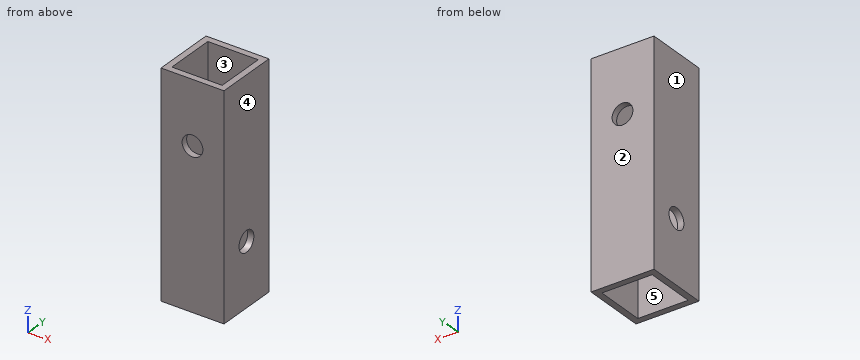
Autodesk Inventor part; units mm, degrees
ref_plane "YZ Plane" through (0, 0, 0) normal (1, 0, 0) x (0, 1, 0)
ref_plane "XZ Plane" through (0, 0, 0) normal (0, 1, 0) x (-1, 0, 0)
ref_plane "XY Plane" through (0, 0, 0) normal (0, 0, 1) x (1, 0, 0)
sketch "スケッチ1" plane through (0, 0, 0) normal (0, 0, 1) x (1, 0, 0)
  line L0 (5, -5) -> (-5, -5)
  line L1 (-5, -5) -> (-5, 5)
  line L2 (-5, 5) -> (5, 5)
  line L3 (5, 5) -> (5, -5)
  line L4 (5, -5) -> (-5, 5) construction
  line L5 (-5, -5) -> (5, 5) construction
  line L6 (4, 4) -> (-4, 4)
  line L7 (-4, 4) -> (-4, -4)
  line L8 (-4, -4) -> (4, -4)
  line L9 (4, -4) -> (4, 4)
  point P0 (0, 0)
  dimension "d0" = 10
  dimension "d1" = 10
  dimension "d2" = 1
extrude "押し出し1" add sketch "スケッチ1" along normal blind 35
sketch "スケッチ2" plane through (5, -5, 0) normal (1, 0, 0) x (0, 0, -1)
  line L0 (-35, 9) -> (-35, 1)
  line L1 (-35, 5) -> (0, 5)
  line L2 (0, 9) -> (0, 1)
  point P0 (-10, 5)
  dimension "d5" = 10
hole "穴1" at (5, 0, 10) direction (-1, 0, 0) diameter 3.3 end through all
sketch "スケッチ3" plane through (-5, 5, 0) normal (0, 1, 0) x (1, 0, 0)
  line L0 (5, 0) -> (5, -35)
  line L1 (0, -35) -> (10, -35)
  line L2 (10, 0) -> (0, 0)
  point P0 (5, -25)
  dimension "d13" = 25
hole "穴2" at (0, 5, 25) direction (0, -1, 0) diameter 3.3 end through all
properties part number "small_kaku_1010_santen_1020"
For this review, take the finished solid that the model builds, in its own axes (mm). Face numbers are marked on the shaded views. A direction names the side the tool comes from. Round coordinates to 2 decimals unless told otherwise and drop trailing zeros. Write each loop counter-clockwise with the first axis right and the second up, starting at its lowest first coordinate (ties: lowest second). Pieces come first, ordered by that corner, then holes. Notation, with made-up numbers: (80.25, 23) -> (130.25, 23) arc R30 cw to (130.25, 50) -> close; hole circle Ø6 at (37.5, 84). An arc over 180 degrees is marked (long way). One line per question, with ' | ' between items. Start each with the question number.
(1) Add section A-A, the plane z = 10. Write out the cut boundary in (x, y), plus the area to 3 significant figures.
(2) Add section B-B, the plane x = 0. Write out the cut boundary in (y, z).
(3) Add section D-D, the plane y = 0. Write out the cut boundary in (x, z).
(4) Add section C-C, the plane y = -2.75. Write out the cut boundary in (x, z).
(5) Tool access review of the marked faces 4 and 5: name each direction out of +Z, -Z, +X, -X, +Y, -Y from which nothing blocks a thin tool from reaching the whole face with its end or side.
(6) Mouldability with a two-part tool opening along Y and no side actions: class the marked faces 1, 2 and 3 as released by +Y, released by -Y, zero draft, split by the parting line, or undercut.
(7) Insertion check: P1, Ø5.5, axis at x = 0, z = 25, coming from the +Y side. The pin has a flat end and moves straight along its axis. Give the tip position at first contact, or say it passes through.
(8) For line 1 along Y through (x, z) = (-2.5, 26); line 2 along Y through (x, z) = (-4.35, 10); line 3 along Z through (x, y) = (0, -4.3), list the stretches that pass through material, from the lowest coordinate up. Write a range as from..to.
Answer list:
1) outline: (-5, -5) -> (5, -5) -> (5, -1.65) -> (4, -1.65) -> (4, -4) -> (-4, -4) -> (-4, -1.65) -> (-5, -1.65) -> close; (-5, 1.65) -> (-4, 1.65) -> (-4, 4) -> (4, 4) -> (4, 1.65) -> (5, 1.65) -> (5, 5) -> (-5, 5) -> close | area: 29.4 mm²
2) outline: (-5, 0) -> (-4, 0) -> (-4, 23.35) -> (-5, 23.35) -> close; (-5, 26.65) -> (-4, 26.65) -> (-4, 35) -> (-5, 35) -> close; (4, 0) -> (5, 0) -> (5, 23.35) -> (4, 23.35) -> close; (4, 26.65) -> (5, 26.65) -> (5, 35) -> (4, 35) -> close
3) outline: (-5, 0) -> (-4, 0) -> (-4, 8.35) -> (-5, 8.35) -> close; (-5, 11.65) -> (-4, 11.65) -> (-4, 35) -> (-5, 35) -> close; (4, 0) -> (5, 0) -> (5, 8.35) -> (4, 8.35) -> close; (4, 11.65) -> (5, 11.65) -> (5, 35) -> (4, 35) -> close
4) outline: (-5, 0) -> (-4, 0) -> (-4, 35) -> (-5, 35) -> close; (4, 0) -> (5, 0) -> (5, 35) -> (4, 35) -> close
5) face 4: +Z, -Z, +X, +Y, -Y | face 5: +Z, -Z
6) face 1: zero draft | face 2: released by +Y | face 3: undercut
7) P1: y = 5
8) line 1: -5..-4, 4..5 | line 2: -5..-1.65, 1.65..5 | line 3: 0..23.35, 26.65..35
